Read the model definition and answer for the solid it produces. Units are mm, in the model's axes. A direction names the side the tool comes from. Coordinates: 2 decimals unless noted, no trailing zeros. Write each loop counter-clockwise with the first axis right and the second up, starting at its lowest first coordinate (ties: lowest second). Pieces come first, ordered by that corner, then holes.
(1) Which of the six approach directions +Z, -Z, +X, -X, +Y, -Y give full straight-line access (tool end or side, diameter ignored) to faces 1 (the cylindrical face through (-2.4, 12.8, 38.3)), 2 (the cylindrical face through (0, 7, -25))?
(2) The part is cut by section B-B, the plane x = 41.5. Determine the outline of the cut face in (y, z).
(3) The part is cut by section C-C, the plane z = 41.5. Determine the outline of the cut face in (x, y).
(4) Given pin 1 (7 mm diameter, centred on x = 41.5, z = 0, fed in from +Y); pin 2 (1 mm diameter, centred on y = 12, z = 9, fed in from -X); pin 3 (9 mm diameter, centred on x = 28.5, z = 31, fed in from +Y); pin 4 (2 mm diameter, centred on y = 3, z = -2, fed in from +X), each flat-ended and moving along its own axis, determine where each tip first touches the part or whether it passes through.
(5) The part is cut by section A-A, the plane x = 0. State how many separate pieces and enclosed holes the cut face has, and give its area (3 significant figures).
(6) Straight lines are drawn through the part: line 1 along X through (y, z) = (6, 0); line 2 along X through (y, z) = (11, 0); line 3 along Z through (x, y) = (31, 12.5). For each, find the intervals that lie inside material, in ascending order.
```python
from build123d import *

# Parameters (mm, degrees)
SKETCH1_R                               = 47.5
SKETCH1_R_2                             = 17.5
SKETCH1_R_3                             = 2.75
SKETCH1_R_4                             = 2.5
BOSS_EXTRUDE1_DEPTH                     = 15
CBORE_FOR_M5_HEX_HEAD_BOLT4_D           = 4.5
CBORE_FOR_M5_HEX_HEAD_BOLT4_CBORE_D     = 8
CBORE_FOR_M5_HEX_HEAD_BOLT4_CBORE_DEPTH = 4.4


with BuildPart() as part:
    # Sketch1 → Boss-Extrude1 (new body)
    with BuildSketch(Plane(origin=(0, 0, 0), x_dir=(1, 0, 0), z_dir=(0, 1, 0))):
        with Locations(Location((0, 0, 0), (0, 0, 270))):
            Circle(SKETCH1_R)
        with Locations(Location((0, 0, 0), (0, 0, 270))):
            Circle(SKETCH1_R_2, mode=Mode.SUBTRACT)
        with Locations(Location((0, 41.5, 0), (0, 0, 270))):
            Circle(SKETCH1_R_3, mode=Mode.SUBTRACT)
        with Locations(Location((29.344931419, 29.344931419, 0), (0, 0, 270))):
            Circle(SKETCH1_R_3, mode=Mode.SUBTRACT)
        with Locations(Location((41.5, 0, 0), (0, 0, 270))):
            Circle(SKETCH1_R_3, mode=Mode.SUBTRACT)
        with Locations(Location((29.344931419, -29.344931419, 0), (0, 0, 270))):
            Circle(SKETCH1_R_3, mode=Mode.SUBTRACT)
        with Locations(Location((0, -41.5, 0), (0, 0, 270))):
            Circle(SKETCH1_R_3, mode=Mode.SUBTRACT)
        with Locations(Location((-29.344931419, -29.344931419, 0), (0, 0, 270))):
            Circle(SKETCH1_R_3, mode=Mode.SUBTRACT)
        with Locations(Location((-41.5, 0, 0), (0, 0, 270))):
            Circle(SKETCH1_R_3, mode=Mode.SUBTRACT)
        with Locations(Location((-29.344931419, 29.344931419, 0), (0, 0, 270))):
            Circle(SKETCH1_R_3, mode=Mode.SUBTRACT)
        with Locations(Location((0, 22.5, 0), (0, 0, 270))):
            Circle(SKETCH1_R_4, mode=Mode.SUBTRACT)
        with Locations(Location((15.909902577, 15.909902577, 0), (0, 0, 270))):
            Circle(SKETCH1_R_4, mode=Mode.SUBTRACT)
        with Locations(Location((22.5, 0, 0), (0, 0, 270))):
            Circle(SKETCH1_R_4, mode=Mode.SUBTRACT)
        with Locations(Location((15.909902577, -15.909902577, 0), (0, 0, 270))):
            Circle(SKETCH1_R_4, mode=Mode.SUBTRACT)
        with Locations(Location((0, -22.5, 0), (0, 0, 270))):
            Circle(SKETCH1_R_4, mode=Mode.SUBTRACT)
        with Locations(Location((-15.909902577, -15.909902577, 0), (0, 0, 270))):
            Circle(SKETCH1_R_4, mode=Mode.SUBTRACT)
        with Locations(Location((-22.5, 0, 0), (0, 0, 270))):
            Circle(SKETCH1_R_4, mode=Mode.SUBTRACT)
        with Locations(Location((-15.909902577, 15.909902577, 0), (0, 0, 270))):
            Circle(SKETCH1_R_4, mode=Mode.SUBTRACT)
    extrude(amount=BOSS_EXTRUDE1_DEPTH)

    # CBORE for M5 Hex Head Bolt4 (through all)
    with Locations(Plane(origin=(0, 15, -41.5), x_dir=(0, 0, 1), z_dir=(0, 1, 0))):
        with Locations((0, 0), (12.155068581, 29.344931419), (41.5, 41.5), (70.844931419, 29.344931419), (83, 0), (70.844931419, -29.344931419), (41.5, -41.5), (12.155068581, -29.344931419)):
            CounterBoreHole(CBORE_FOR_M5_HEX_HEAD_BOLT4_D / 2, CBORE_FOR_M5_HEX_HEAD_BOLT4_CBORE_D / 2, CBORE_FOR_M5_HEX_HEAD_BOLT4_CBORE_DEPTH)


solid = part.part
```
Computed:
1. face 1: +Y
1. face 2: +Y, -Y
2. outline: (0, -23.11) - (15, -23.11) - (15, -4) - (10.6, -4) - (10.6, -2.75) - (0, -2.75) - close; (0, 2.75) - (10.6, 2.75) - (10.6, 4) - (15, 4) - (15, 23.11) - (0, 23.11) - close
3. outline: (-23.11, 0) - (-2.75, 0) - (-2.75, 10.6) - (-4, 10.6) - (-4, 15) - (-23.11, 15) - close; (2.75, 0) - (23.11, 0) - (23.11, 15) - (4, 15) - (4, 10.6) - (2.75, 10.6) - close
4. pin 1: stops at y = 10.6
4. pin 2: stops at x = -46.73
4. pin 3: stops at y = 15
4. pin 4: stops at x = 47.49
5. separate pieces: 6
5. enclosed holes: 0
5. area: 563 mm2
6. line 1: x = -47.5 to -44.25, -38.75 to -25, -20 to -17.5, 17.5 to 20, 25 to 38.75, 44.25 to 47.5
6. line 2: x = -47.5 to -45.5, -37.5 to -25, -20 to -17.5, 17.5 to 20, 25 to 37.5, 45.5 to 47.5
6. line 3: z = -35.99 to -32.99, -25.7 to 25.7, 32.99 to 35.99
